The listing builds one solid part. Answer for the finished solid, in the listing's coordinates (mm). A direction names the side the tool comes from. Coordinates: 2 decimals unless noted, no trailing zeros. Order: outer loops, then holes, each group sorted by start corner. A loop starts at its lowest first (then second) coordinate and runs counter-clockwise, first axis right, second up. Notation, with made-up numbers: (-2, 10) -> (40, 10) arc R24 ccw to (40, 25) -> close; hole circle Ø5 at (-22, 45.25). An arc over 180 degrees is marked (long way). Write item = value, one per line.
from build123d import *
from build123d.topology import SkipClean

# Parameters (mm, degrees)
SKETCH1_R                = 1.5
BOSS_EXTRUDE1_DEPTH      = 2.5
BOSS_EXTRUDE2_DEPTH      = 6.9
BOSS_EXTRUDE2_DEPTH_BACK = 2.5
SKETCH2_R                = 4.5
SKETCH2_R_2              = 1.5
SKETCH4_R                = 2.5
CUT_EXTRUDE1_DEPTH       = 2
BOSS_EXTRUDE3_START      = 0.75
SKETCH5_R                = 4.5
SKETCH5_R_2              = 2.5
BOSS_EXTRUDE3_DEPTH      = 0.75
BOSS_EXTRUDE4_DEPTH      = 2.5
CUT_EXTRUDE2_REACH       = 80.314
SKETCH7_W                = 7
SKETCH7_H                = 16.5
SKETCH7_W_2              = 16
SKETCH7_H_2              = 8
CUT_EXTRUDE3_REACH       = 82.041
SKETCH9_W                = 2.5
SKETCH9_H                = 22.388822383
BOSS_EXTRUDE5_DEPTH      = 12.5
FILLET2_R                = 1
FILLET3_R                = 4
CUT_EXTRUDE4_DEPTH       = 74.103052287
CUT_EXTRUDE4_DEPTH_BACK  = 74.103052287
SKETCH10_W               = 78.235731334
SKETCH10_H               = 6.290045588
SKETCH11_W               = 14.9
SKETCH11_H               = 2.5
BOSS_EXTRUDE6_DEPTH      = 12.5
BOSS_EXTRUDE7_DEPTH      = 2.5
SKETCH14_R               = 1.5
CUT_EXTRUDE5_DEPTH       = 2.5


with BuildPart() as part:
    # Sketch1 → Boss-Extrude1 (new body)
    with BuildSketch(Plane(origin=(0, 0, 0), x_dir=(0, 0, -1), z_dir=(1, 0, 0))):
        with BuildLine():
            Line((0, 12.5), (34.45, 12.5))
            Line((34.45, 12.5), (34.45, -12.5))
            Line((34.45, -12.5), (0, -12.5))
            ThreePointArc((0, -12.5), (-12.5, 0), (0, 12.5))
        make_face()
        Circle(SKETCH1_R, mode=Mode.SUBTRACT)
    extrude(amount=BOSS_EXTRUDE1_DEPTH)

    # Sketch2 → Boss-Extrude2 (add, two sides: drawn at the far end of the back side and taken through both)
    with BuildSketch(Plane.ZY.offset(-BOSS_EXTRUDE2_DEPTH_BACK)):
        Circle(SKETCH2_R)
        Circle(SKETCH2_R_2, mode=Mode.SUBTRACT)
    extrude(amount=BOSS_EXTRUDE2_DEPTH + BOSS_EXTRUDE2_DEPTH_BACK)

    # Sketch4 → Cut-Extrude1 (cut)
    with BuildSketch(Plane(origin=(2.5, 0, 0), x_dir=(0, 0, -1), z_dir=(1, 0, 0))):
        Circle(SKETCH4_R)
    extrude(amount=-CUT_EXTRUDE1_DEPTH, mode=Mode.SUBTRACT)

    # Sketch5 → Boss-Extrude3 (add)
    with SkipClean():  # the faces are left unmerged after this step: merging them gives an invalid solid
        with BuildSketch(Plane(origin=(2.5, 0, 0), x_dir=(0, 0, -1), z_dir=(1, 0, 0)).offset(BOSS_EXTRUDE3_START)):
            with Locations(Location((0, 0, 0), (0, 0, 180))):
                Circle(SKETCH5_R)
            Circle(SKETCH5_R_2, mode=Mode.SUBTRACT)
        extrude(amount=-BOSS_EXTRUDE3_DEPTH)

    # Sketch6 → Boss-Extrude4 (add)
    with SkipClean():  # the faces are left unmerged after this step: merging them gives an invalid solid
        with BuildSketch(Plane(origin=(0, 0, -34.45), x_dir=(-1, 0, 0), z_dir=(0, 0, -1))):
            Polygon((-8.812505246, 36.25), (53.321583376, 36.25), (53.321583376, -36.25), (6.25, -36.25), (-19.178416624, -36.25), (-19.178416624, 36.25), align=None)
        extrude(amount=-BOSS_EXTRUDE4_DEPTH)
    add(part.part.scale(1), mode=Mode.REPLACE)  # the faces are merged on a copy

    # Sketch7 → Cut-Extrude2 (cut, up to next)
    with BuildSketch(Plane.XY.offset(-31.95), mode=Mode.PRIVATE) as cut_extrude2_sk1:
        with Locations((-1.711858899, -11.632438111)):
            Rectangle(SKETCH7_W, SKETCH7_H)
    cut_extrude2_tool1 = extrude(cut_extrude2_sk1.sketch, amount=-CUT_EXTRUDE2_REACH, mode=Mode.PRIVATE) & part.part
    # Sketch7 → Cut-Extrude2 (cut, up to next)
    with BuildSketch(Plane.XY.offset(-31.95), mode=Mode.PRIVATE) as cut_extrude2_sk2:
        with Locations((-16.5, 0)):
            Rectangle(SKETCH7_W_2, SKETCH7_H_2)
    cut_extrude2_tool2 = extrude(cut_extrude2_sk2.sketch, amount=-CUT_EXTRUDE2_REACH, mode=Mode.PRIVATE) & part.part
    add(cut_extrude2_tool1.solids().sort_by_distance((-1.711859, -11.632438, -31.95))[0], mode=Mode.SUBTRACT)
    add(cut_extrude2_tool2.solids().sort_by_distance((-16.5, 0, -31.95))[0], mode=Mode.SUBTRACT)

    # Sketch9 → Cut-Extrude3 (cut, up to next)
    with BuildSketch(Plane.XZ.offset(12.5), mode=Mode.PRIVATE) as cut_extrude3_sk1:
        with Locations((1.25, -20.755588809)):
            Rectangle(SKETCH9_W, SKETCH9_H)
    cut_extrude3_tool1 = extrude(cut_extrude3_sk1.sketch, amount=-CUT_EXTRUDE3_REACH, mode=Mode.PRIVATE) & part.part
    add(cut_extrude3_tool1.solids().sort_by_distance((1.25, -12.5, -20.755589))[0], mode=Mode.SUBTRACT)


with BuildPart() as cut_extrude3_piece_1:
    # of the separate pieces the step leaves, piece 1, a body of its own (cut_extrude3_pieces)
    add(part.part.solids().sort_by_distance((-53.321583376, 36.25, -31.95))[0])



with BuildPart() as cut_extrude3_piece_2:
    # of the separate pieces the step leaves, piece 2, a body of its own (cut_extrude3_pieces)
    add(part.part.solids().sort_by_distance((0, 12.5, 0))[0])


with BuildPart() as cut_extrude3_piece_1_1:
    add(cut_extrude3_piece_1.part)

    add(cut_extrude3_piece_2.part)  # Boss-Extrude5 merges Cut-Extrude3 piece 2
    # Sketch8 → Boss-Extrude5 (add, symmetric)
    with BuildSketch(Plane(origin=(0, 0, 0), x_dir=(1, 0, 0), z_dir=(0, 1, 0))):
        with BuildLine():
            Line((0, 7.729605828), (2.5, 7.729605828))
            Line((2.5, 7.729605828), (2.5, 10.229605828))
            ThreePointArc((2.5, 10.229605828), (1.573627862, 16.099871922), (-1.115452176, 21.399592472))
            ThreePointArc((-1.115452176, 21.399592472), (-3.053519862, 25.219195088), (-3.721172696, 29.45))
            Line((-3.721172696, 29.45), (-3.721172696, 31.95))
            Line((-3.721172696, 31.95), (-6.221172696, 31.95))
            Line((-6.221172696, 31.95), (-6.221172696, 28.45))
            ThreePointArc((-6.221172696, 28.45), (-5.429444077, 23.92831405), (-3.148463103, 19.944646916))
            ThreePointArc((-3.148463103, 19.944646916), (-0.81124762, 15.862767844), (0, 11.229605828))
            Line((0, 11.229605828), (0, 7.729605828))
        make_face()
    extrude(amount=BOSS_EXTRUDE5_DEPTH, both=True)

    # Fillet2
    fillet2_edges = [cut_extrude3_piece_1_1.edges().sort_by_distance(p)[0] for p in [
        (-8.5, 4, -33.2),
        (-8.5, -4, -33.2),
        (-24.5, -4, -33.2),
        (-24.5, 4, -33.2),
        (-5.211858899, -19.882438111, -33.2),
        (-5.211858899, -3.382438111, -33.2),
        (1.788141101, -3.382438111, -33.2),
        (1.788141101, -19.882438111, -33.2),
    ]]
    fillet(fillet2_edges, radius=FILLET2_R)

    # Fillet3
    fillet3_edges = [cut_extrude3_piece_1_1.edges().sort_by_distance(p)[0] for p in [
        (19.178416624, 36.25, -33.2),
        (-53.321583376, 36.25, -33.2),
        (-53.321583376, -36.25, -33.2),
        (19.178416624, -36.25, -33.2),
    ]]
    fillet(fillet3_edges, radius=FILLET3_R)

    # Sketch10 → Cut-Extrude4 (cut, two sides: drawn at the far end of the back side and taken through both)
    with SkipClean():  # the faces are left unmerged after this step: merging them gives an invalid solid
        with BuildSketch(Plane(origin=(0, 0, 0), x_dir=(1, 0, 0), z_dir=(0, 1, 0)).offset(-CUT_EXTRUDE4_DEPTH_BACK)):
            with Locations((-17.391929865, 35.095022794)):
                Rectangle(SKETCH10_W, SKETCH10_H)
        extrude(amount=CUT_EXTRUDE4_DEPTH + CUT_EXTRUDE4_DEPTH_BACK, mode=Mode.SUBTRACT)

    # Sketch11 → Boss-Extrude6 (add, symmetric)
    with BuildSketch(Plane(origin=(0, 0, 0), x_dir=(1, 0, 0), z_dir=(0, 1, 0))):
        with Locations((3.728827304, 30.7)):
            Rectangle(SKETCH11_W, SKETCH11_H)
    boss_extrude6 = extrude(amount=BOSS_EXTRUDE6_DEPTH, both=True)

    # Sketch13 → Boss-Extrude7 (add)
    with BuildSketch(Plane(origin=(0, 0, -31.95), x_dir=(-1, 0, 0), z_dir=(0, 0, -1))):
        with BuildLine():
            Line((-11.178827304, 12.5), (3.821172696, 12.5))
            Line((3.821172696, 12.5), (3.821172696, 28.75))
            Line((3.821172696, 28.75), (3.821172696, 36.25))
            Line((3.821172696, 36.25), (-3.678827304, 36.25))
            Line((-3.678827304, 36.25), (-7.178827304, 36.25))
            ThreePointArc((-7.178827304, 36.25), (-10.007254429, 35.078427125), (-11.178827304, 32.25))
            Line((-11.178827304, 32.25), (-11.178827304, 28.75))
            Line((-11.178827304, 28.75), (-11.178827304, 12.5))
        make_face()
    boss_extrude7 = extrude(amount=-BOSS_EXTRUDE7_DEPTH)

    # Mirror1: Boss-Extrude6, Boss-Extrude7 across plane
    add(boss_extrude6.mirror(Plane.ZX))
    add(boss_extrude7.mirror(Plane.ZX))

    # Sketch14 → Cut-Extrude5 (cut)
    with BuildSketch(Plane(origin=(0, 0, -31.95), x_dir=(-1, 0, 0), z_dir=(0, 0, -1))):
        with Locations((-3.678827304, 28.75)):
            Circle(SKETCH14_R)
    cut_extrude5 = extrude(amount=-CUT_EXTRUDE5_DEPTH, mode=Mode.SUBTRACT)

    # Mirror2: Cut-Extrude5 across plane
    add(cut_extrude5.mirror(Plane.ZX), mode=Mode.SUBTRACT)


solid = cut_extrude3_piece_1_1.part
Q1. Find the intervals of material crossed by line 1 along Y through (x, z) = (-2.25, 0); line 2 along Z through (x, y) = (10, 0); line 3 along X through (y, z) = (10, 2), in increasing order.
The answers:
line_1 = -4.5 to -1.5, 1.5 to 4.5
line_2 = -31.95 to -29.45
line_3 = 0 to 2.5
Q2. Each of these flat-tipped pins is pushed along its axis until it touches: pin 1 Ø1.5 at (y, z) = (10.5, -5) entering from -X; pin 2 Ø7 at (y, z) = (-1, 2) entering from +X; pin 3 Ø2.5 at (x, z) = (-3, -14) entering from -Y; pin 4 Ø3.5 at (y, z) = (0, 0) entering from +X. Where does it stop, or does it pass through?
The answers:
pin_1 = 0
pin_2 = 3.25
pin_3 = through
pin_4 = 0.5
Q3. The mould has two halves that part along X. Classify faces 4 (the face through (-3.4, 4.46, -0.59)), 5 (the face through (-3.821, -24, -31)), 6 (the face through (3.874, 30.237, -30.718)): released by +X, released by -X, zero draft, split by the parting line, or undercut.
The answers:
face_4 = zero draft
face_5 = released by -X
face_6 = undercut
Q4. Section A-A, the plane y = -28.75 is taken. Give the vertices of the cut face in (x, z), plus the area to 3 significant figures.
The answers:
outline = (-3.82, -31.95) -> (2.18, -31.95) -> (2.18, -29.45) -> (-3.82, -29.45) -> close; (5.18, -31.95) -> (11.18, -31.95) -> (11.18, -29.45) -> (5.18, -29.45) -> close
area = 30.0 mm2
Q5. Section B-B, the plane x = 4.25 is taken. Give the vertices of the cut face in (y, z), plus the area to 3 significant figures.
The answers:
outline = (-36.25, -31.95) -> (-30.14, -31.95) -> (-30.14, -29.45) -> (-36.25, -29.45) -> close; (-27.36, -31.95) -> (27.36, -31.95) -> (27.36, -29.45) -> (-27.36, -29.45) -> close; (30.14, -31.95) -> (36.25, -31.95) -> (36.25, -29.45) -> (30.14, -29.45) -> close
area = 167 mm2
Q6. Section C-C, the plane x = -5.25 is taken. Give the vertices of the cut face in (y, z), plus the area to 3 significant figures.
The answers:
outline = (-12.5, -31.95) -> (12.5, -31.95) -> (12.5, -23.46) -> (-12.5, -23.46) -> close; circle Ø9 at (0, 0); hole circle Ø3 at (0, 0)
area = 269 mm2
Q7. Section D-D, the plane y = -3.5 is taken. Give the vertices of the cut face in (x, z), plus the area to 3 significant figures.
The answers:
outline = (-6.9, -2.83) -> (0, -2.83) -> (0, -11.23) arc R13.64 cw to (-3.15, -19.94) arc R13.31 ccw to (-6.22, -28.45) -> (-6.22, -31.95) -> (11.18, -31.95) -> (11.18, -29.45) -> (-3.72, -29.45) arc R13.74 cw to (-1.12, -21.4) arc R19.06 ccw to (2.5, -10.23) -> (2.5, -2.83) -> (3.25, -2.83) -> (3.25, 2.83) -> (2.5, 2.83) -> (2.5, 12) -> (0, 12) -> (0, 2.83) -> (-6.9, 2.83) -> close
area = 194 mm2
Q8. A tool of negligible diameter and unlimited length cuts with its end or side. For faces 1 (the face through (3.25, 2, 2)), 2 (the face through (0, 0, -5)), 3 (the face through (-0.83, 0.18, -15.92)), from which of +Z, -Z, +X, -X, +Y, -Y can it reach the whole face along a straight path? Write none if from no direction.
The answers:
face_1 = +Z, +X, +Y, -Y
face_2 = -X
face_3 = -X, +Y, -Y
